```python
from build123d import *

# Parameters (mm, degrees)
ESBO_O1_R                = 20
RESSALTO_EXTRUS_O1_DEPTH = 20
FILETE1_R                = 10
ESBO_O3_R                = 12.5
RESSALTO_EXTRUS_O2_DEPTH = 20
ESBO_O6_R                = 3
CORTE_EXTRUS_O1_DEPTH    = 30


with BuildPart() as part:
    # Esboço1 → Ressalto-extrusão1 (new body)
    with BuildSketch(Plane.XY):
        Circle(ESBO_O1_R)
    extrude(amount=RESSALTO_EXTRUS_O1_DEPTH)

    # Filete1
    filete1_edges = [part.edges().sort_by_distance(p)[0] for p in [
        (-20, 0, 20),
    ]]
    fillet(filete1_edges, radius=FILETE1_R)

    # Esboço3 → Ressalto-extrusão2 (add)
    with BuildSketch(Plane(origin=(0, 0, 0), x_dir=(-1, 0, 0), z_dir=(0, 0, -1))):
        Circle(ESBO_O3_R)
    extrude(amount=RESSALTO_EXTRUS_O2_DEPTH)

    # Esboço6 → Corte-extrusão1 (cut)
    with BuildSketch(Plane(origin=(0, 0, -20), x_dir=(-1, 0, 0), z_dir=(0, 0, -1))):
        Circle(ESBO_O6_R)
    extrude(amount=-CORTE_EXTRUS_O1_DEPTH, mode=Mode.SUBTRACT)


solid = part.part
```
Model file for the job. Use its own axes, mm. A direction names the side the tool comes from. Give positions to 0.01 mm unless a question says otherwise; leave off trailing zeros. Order: outer loops, then holes, each group sorted by start corner. A loop starts at its lowest first (then second) coordinate and runs counter-clockwise, first axis right, second up.
1) 3-axis set-ups, long thin cutter, end or side, ignore diameter. For faces 1 (the flat face through (0, 0, 20)), 2 (the cylindrical face through (3, 0, -5)): which of +Z, -Z, +X, -X, +Y, -Y reach the whole face in a straight line?
2) Saw through at B-B, the plane z = 8. Write the cut outline in (x, y), then the cut area to 3 significant figures.
3) Mould opens along X. For faces 3 (the flat face through (0, 0, 10)), 4 (the cylindrical face through (-11.923, 3.755, -9.86)), 5 (the flat face through (-3, -3, -20)) say: +X half, -X half, draft (parallel to the pull), parting line (faces both ways), or undercut.
4) Saw through at A-A, the plane z = -6.5. Write the cut outline in (x, y).
5) Wall check: probe 1 along Y at (x, z) = (0, -0.75); probe 2 along X at (y, z) = (2, -1). Give the ranges that are in metal, low to high.
6) Pin check, flat tips, straight feed: pin 1 (2 mm diameter, centred on x = -2, z = 15, fed in from +Y); pin 2 (2 mm diameter, centred on y = -7.5, z = 10.5, fed in from -X); pin 3 (3 mm diameter, centred on x = 1, y = 1, fed in from -Z); pin 4 (5 mm diameter, centred on x = -15.5, z = -6.5, fed in from -Y). Stop position of each tip, or through.
Computed:
1. face 1: +Z, +X, -X, +Y, -Y
1. face 2: -Z
2. outline: circle Ø40 at (0, 0); hole circle Ø6 at (0, 0)
2. area: 1,230 mm2
3. face 3: undercut
3. face 4: parting line
3. face 5: draft
4. outline: circle Ø25 at (0, 0); hole circle Ø6 at (0, 0)
5. probe 1: y = -12.5 to -3, 3 to 12.5
5. probe 2: x = -12.34 to -2.24, 2.24 to 12.34
6. pin 1: stops at y = 19.07
6. pin 2: stops at x = -18.9
6. pin 3: stops at z = 10
6. pin 4: passes through
